Part model, mm, in its own coordinate system. A direction names the side the tool comes from. Coordinates: 2 decimals unless noted, no trailing zeros. Write each loop counter-clockwise with the first axis right and the second up, starting at its lowest first coordinate (ties: lowest second). Pieces come first, ordered by that corner, then holes. Notation, with made-up numbers: (4, 30.25) - (51, 30.25) arc R17 cw to (51, 45.25) - close; hole circle Ø2 at (-21.75, 42). An arc over 180 degrees is marked (long way). Write each question's results on one line, items separated by ' | '.
from build123d import *

# Parameters (mm, degrees)
F1_DEPTH = 2400
F2_T     = -2.5


with BuildPart() as f1:
    # F0 (on Right) → F1 (new body)
    with BuildSketch(Plane.YZ):
        Polygon((1054.663021, -663.515762), (415.721765, 352.237196), (0, 352.237196), (-430.056426, -241.650613), (-430.056426, -534.498729), (-260.08166, -663.515762), align=None)
    extrude(amount=F1_DEPTH)

    # F2
    f2_openings = [f1.faces().sort_by_distance(p)[0] for p in [
        (1200, 735.192393, -155.639283),
    ]]
    offset(amount=F2_T, openings=f2_openings)


solid = f1.part
(1) Saw through at B-B on x = 391.5. Write the cut outline in (y, z), then the cut area to 3 significant figures.
Return value:
outline: (-430.06, -534.5) - (-260.08, -663.52) - (1054.66, -663.52) - (1053.09, -661.02) - (-259.24, -661.02) - (-427.56, -533.26) - (-427.56, -242.46) - (1.28, 349.74) - (417.29, 349.74) - (415.72, 352.24) - (0, 352.24) - (-430.06, -241.65) - close | area: 7,410 mm^2
(2) Flat gauge pins, fed straight in: P1, Ø5, axis at x = 1615.5, y = 562, coming from the +Z side; P2, Ø10, axis at x = 1664.5, z = -44, coming from the +Y side; P3, Ø5, axis at x = 605, y = -162, coming from the +Z side. Where does each tip first touch, or does it go through?
Return value:
P1: stops at z = -661.02 | P2: stops at y = -280.22 | P3: stops at z = 131.98
(3) Two-plate mould, pull along X, no slides. Class faces 1 (the flat face through (1183.2, -212.02, 59.45)), 2 (the flat face through (1183, 212, 349.737)), 3 (the flat face through (2400, 302, -261)), 4 (the flat face through (1183, 388, -661.016)): released by +X, released by -X, zero draft, split by the parting line, or undercut.
Return value:
face 1: zero draft | face 2: undercut | face 3: released by +X | face 4: undercut
(4) Saw through at C-C on z = 228. Write the cut outline in (x, y), then the cut area to 3 significant figures.
Return value:
outline: (0, -89.96) - (2400, -89.96) - (2400, 493.87) - (2397.5, 493.87) - (2397.5, -86.88) - (2.5, -86.88) - (2.5, 493.87) - (0, 493.87) - close | area: 10,300 mm^2
(5) Saw through at D-D on y = 865. Write the cut outline in (x, z).
Return value:
outline: (0, -663.52) - (2400, -663.52) - (2400, -362) - (2397.5, -362) - (2397.5, -661.02) - (2.5, -661.02) - (2.5, -362) - (0, -362) - close
(6) Saw through at A-A on y = 323.5. Write the cut outline in (x, z).
Return value:
outline: (0, -663.52) - (2400, -663.52) - (2400, 352.24) - (0, 352.24) - close; hole (2.5, -661.02) - (2397.5, -661.02) - (2397.5, 349.74) - (2.5, 349.74) - close
(7) Wall check: line 1 (Z direction, x = 174.5, y = 158); line 2 (X direction, y = -119.5, z = -596); line 3 (Z direction, x = 203, y = 642). Give the ranges that are in metal, low to high. Write a range as from..to.
Return value:
line 1: z = -663.52..-661.02, 349.74..352.24 | line 2: x = 0..2.5, 2397.5..2400 | line 3: z = -663.52..-661.02
(8) 3-axis set-ups, long thin cutter, end or side, ignore diameter. For faces 5 (the flat face through (2.5, 302, -261)), 6 (the flat face through (1183, 211, 352.237)): which of +Z, -Z, +X, -X, +Y, -Y reach the whole face in a straight line?
Return value:
face 5: +Y | face 6: +Z, +X, -X, +Y, -Y
